Design review of the part shown in the three views and the two pictorial views. Dimensions are in mm from the part's minimum x, y and z. A direction names the side the tool comes from. Round coordinates to 2 decimals unless told otherwise and drop trailing zeros. Loops run counter-clockwise (first coordinate to the right, second up) from the corner with the lowest first, then second, coordinate; pieces in that order, holes last.
1. Consider section C-C on x = 20. State the section outline as (y, z) points.
2. Consider section A-A on z = 22.5. State the section outline as (x, y) points.
3. Consider section D-D on x = 1.5. State the section outline as (y, z) points.
4. Clearance check with flat-ended pins moving along their axes: pin 1 Ø6 at (x, y) = (12.5, 34.5) entering from +Z; pin 2 Ø8 at (y, z) = (25.5, 21) entering from +X; pin 3 Ø3 at (x, z) = (15.5, 33.5) entering from +Y. State where each tip first meets the part, or that it passes through.
5. Tool access review of the marked faces 1 and 2: name each direction out of +Z, -Z, +X, -X, +Y, -Y from which nothing blocks a thin tool from reaching the whole face with its end or side.
6. To check wall thickness, follow line 1 along Y through (x, z) = (15.25, 22.5); line 2 along X through (y, z) = (13, 11.5); line 3 along Z through (x, y) = (11.5, 20.5). State the ranges of each line that lie inside material, in increasing order.
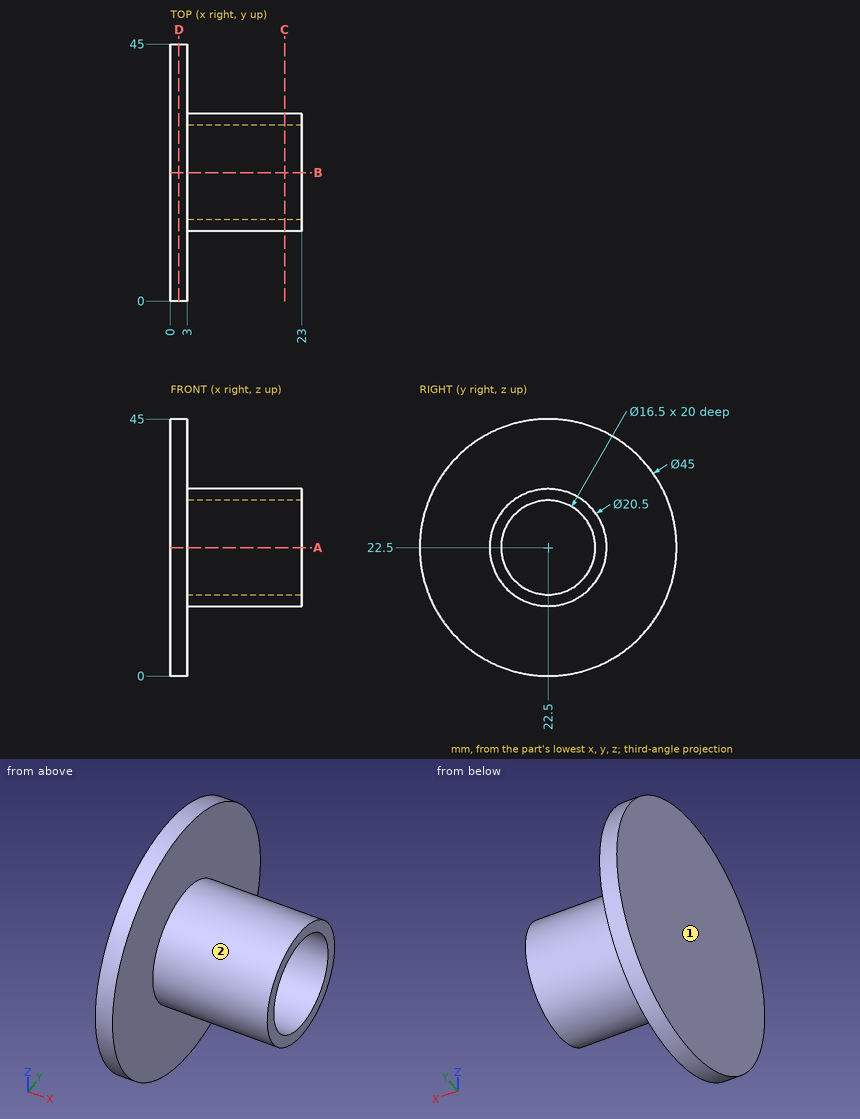
Resolved:
1. outline: circle Ø20.5 at (22.5, 22.5); hole circle Ø16.5 at (22.5, 22.5)
2. outline: (0, 0) - (3, 0) - (3, 12.25) - (23, 12.25) - (23, 14.25) - (3, 14.25) - (3, 30.75) - (23, 30.75) - (23, 32.75) - (3, 32.75) - (3, 45) - (0, 45) - close
3. outline: circle Ø45 at (22.5, 22.5)
4. pin 1: stops at z = 27.41
4. pin 2: stops at x = 3
4. pin 3: stops at y = 26.35
5. face 1: +Z, -Z, -X, +Y, -Y
5. face 2: +X
6. line 1: y = 12.25 to 14.25, 30.75 to 32.75
6. line 2: x = 0 to 3
6. line 3: z = 12.45 to 14.5, 30.5 to 32.55
